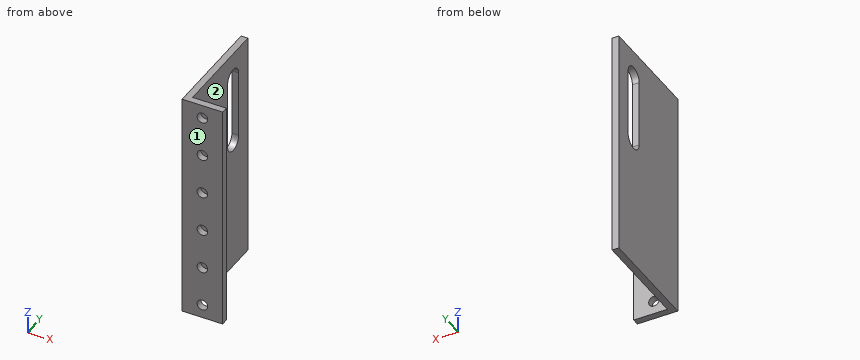
from build123d import *

# Parameters (mm, degrees)
SKETCH1_W           = 3.175
SKETCH1_H           = 47.625
SKETCH1_H_2         = 3.175
SKETCH1_W_2         = 15.875
BOSS_EXTRUDE1_DEPTH = 107.95
SKETCH2_R           = 2.4892
CUT_EXTRUDE1_DEPTH  = 107.95
CUT_EXTRUDE2_DEPTH  = 165.1


with BuildPart() as part:
    # Sketch1 → Boss-Extrude1 (new body)
    with BuildSketch(Plane.XY):
        with Locations((1.5875, 26.9875)):
            Rectangle(SKETCH1_W, SKETCH1_H)
        with Locations((1.5875, 1.5875)):
            Rectangle(SKETCH1_W, SKETCH1_H_2)
        with Locations((11.1125, 1.5875)):
            Rectangle(SKETCH1_W_2, SKETCH1_H_2)
    extrude(amount=BOSS_EXTRUDE1_DEPTH)

    # Sketch2 → Cut-Extrude1 (cut)
    with BuildSketch(Plane(origin=(0, 3.175, 0), x_dir=(1, 0, 0), z_dir=(0, 1, 0))):
        with Locations(Location((9.525, -6.35, 0), (0, 0, 270))):
            Circle(SKETCH2_R)
        with Locations(Location((9.525, -25.4, 0), (0, 0, 270))):
            Circle(SKETCH2_R)
        with Locations(Location((9.525, -44.45, 0), (0, 0, 270))):
            Circle(SKETCH2_R)
        with Locations(Location((9.525, -63.5, 0), (0, 0, 270))):
            Circle(SKETCH2_R)
        with Locations(Location((9.525, -82.55, 0), (0, 0, 270))):
            Circle(SKETCH2_R)
        with Locations(Location((9.525, -101.6, 0), (0, 0, 270))):
            Circle(SKETCH2_R)
    extrude(amount=-CUT_EXTRUDE1_DEPTH, mode=Mode.SUBTRACT)

    # Sketch3 → Cut-Extrude2 (cut)
    with BuildSketch(Plane.ZY):
        with BuildLine():
            Line((63.5, 42.8625), (95.25, 42.8625))
            ThreePointArc((95.25, 42.8625), (100.0125, 38.1), (95.25, 33.3375))
            Line((95.25, 33.3375), (63.5, 33.3375))
            ThreePointArc((63.5, 33.3375), (58.7375, 38.1), (63.5, 42.8625))
        make_face()
    extrude(amount=-CUT_EXTRUDE2_DEPTH, mode=Mode.SUBTRACT)


solid = part.part
Build history of the part. All positions in model axes, mm. Face numbers are marked on the shaded views. A direction names the side the tool comes from. Coordinates: 2 decimals unless noted, no trailing zeros. Write each loop counter-clockwise with the first axis right and the second up, starting at its lowest first coordinate (ties: lowest second). Pieces come first, ordered by that corner, then holes.
(1) Cut at A-A on z = 44.45. List the corners of the cut face in (x, y) (3 decimals).
(2) 3-axis set-ups, long thin cutter, end or side, ignore diameter. For the marked faces 1 and 2: which of +Z, -Z, +X, -X, +Y, -Y reach the whole face in a straight line?
(3) Pin check, flat tips, straight feed: pin 1 Ø5 at (y, z) = (44.5, 78) entering from +X (3 decimals); pin 2 Ø6 at (x, z) = (17, 37) entering from +Y (3 decimals); pin 3 Ø8 at (x, y) = (4, 35) entering from -Z. Stop position of each tip, or through.
(4) Drill centre lines: line 1 (Y direction, x = 2.5, z = 82); line 2 (Y direction, x = 5.75, z = 42) (3 decimals). Where is each one in solid material? Low to high.
Working result:
1. outline: (0, 0) - (7.036, 0) - (7.036, 3.175) - (3.175, 3.175) - (3.175, 50.8) - (0, 50.8) - close; (12.014, 0) - (19.05, 0) - (19.05, 3.175) - (12.014, 3.175) - close
2. face 1: +Z, -Z, +X, -X, -Y
2. face 2: +Z, -Z, +X, +Y
3. pin 1: stops at x = 3.175
3. pin 2: stops at y = 3.175
3. pin 3: stops at z = 0
4. line 1: y = 0 to 33.34, 42.86 to 50.8
4. line 2: y = 0 to 3.175
